Autodesk Inventor part; units mm, degrees
ref_plane "YZ Plane" through (0, 0, 0) normal (1, 0, 0) x (0, 1, 0)
ref_plane "XZ Plane" through (0, 0, 0) normal (0, 1, 0) x (-1, 0, 0)
ref_plane "XY Plane" through (0, 0, 0) normal (0, 0, 1) x (1, 0, 0)
sketch "草图1" plane through (0, 0, 0) normal (0, 0, 1) x (1, 0, 0)
  line L0 (-18, -13) -> (18, -13)
  line L1 (18, -13) -> (18, 13)
  line L2 (18, 13) -> (-18, 13)
  line L3 (-18, 13) -> (-18, -13)
  point P0 (0, 0)
  point P1 (0, 13)
  point P2 (-18, 0)
  dimension "d0" = 36
  dimension "d1" = 26
extrude "拉伸1" add sketch "草图1" along normal mid plane 60
sketch "草图2" plane through (-18, -13, -30) normal (0, -1, 0) x (1, 0, 0)
  line L0 (0, 0) -> (0, 60)
  line L1 (36, 60) -> (0, 60)
  line L2 (36, 0) -> (0, 0)
  arc A0 (20.5, -4) -> (18, -1.5) centre (18, -4) ccw
  line L3 (21.3793, -7) -> (20.5, -7)
  line L4 (20.5, -7) -> (20.5, -4)
  line L5 (23.1821, -5.866) -> (26, 0)
  arc A1 (18, -1.5) -> (15.5, -4) centre (18, -4) ccw
  line L6 (14.6207, -7) -> (15.5, -7)
  line L7 (15.5, -7) -> (15.5, -4)
  line L8 (12.8179, -5.866) -> (10, 0)
  arc A2 (21.3793, -7) -> (23.1821, -5.866) centre (21.3793, -5) ccw
  arc A3 (12.8179, -5.866) -> (14.6207, -7) centre (14.6207, -5) ccw
  point P0 (18, 30)
  point P1 (22.6373, 30)
  point P2 (0, 30)
  point P3 (18, 0)
  point P4 (18, 30)
  point P5 (0, 30)
  point P6 (18, 0)
  point P7 (10, 0)
  dimension "d6" = 5
  dimension "d9" = 2
extrude "拉伸2" add sketch "草图2" against normal blind 2
mirror "镜像1" about plane through (0, 0, 0) normal (0, 0, 1) of "拉伸2"
properties part number "DC_DC_POWER"
The listing builds one solid part. Answer for the finished solid, in the listing's coordinates (mm). A direction names the side the tool comes from. Give positions to 0.01 mm unless a question says otherwise; leave off trailing zeros. Loops run counter-clockwise (first coordinate to the right, second up) from the corner with the lowest first, then second, coordinate; pieces in that order, holes last. Notation, with made-up numbers: M 2,-1.5 L 37,-1.5 A22 cw 37,35.5 Z; hole C 63.25,43 d9. An arc over 180 degrees is marked long. One line per item, written item: value.
1. For faces 4 (the face through (0, -11, -31)), 5 (the face through (2.5, -12, -36)), 6 (the face through (0, -11, 31)), 7 (the face through (-2.5, -12, 35)), determine the directions among +Z, -Z, +X, -X, +Y, -Y from which every point of the face is accessible in a straight line to the end or side of a thin tool.
Found:
face 4: -Z, +X, -X, +Y
face 5: -Z, +Y, -Y
face 6: +Z, +X, -X, +Y
face 7: +Z, +Y, -Y
2. Each of these flat-tipped pins is pushed along its axis until it touches: P1, Ø8, axis at x = 13.5, y = -9.5, coming from the -Z side; P2, Ø2, axis at y = -12, z = 35.5, coming from the -X side; P3, Ø12, axis at x = -14, y = 8, coming from the +Z side. Where does it stop, or does it pass through?
Found:
P1: z = -30
P2: x = -5.84
P3: z = 30
3. Section C-C on x = -6 is taken. Determine the outline of the cut face in (y, z).
Found:
outline: M -13,-34.16 L -11,-34.16 L -11,-30 L 13,-30 L 13,30 L -11,30 L -11,34.16 L -13,34.16 Z
4. Section D-D on x = 11 is taken. Determine the outline of the cut face in (y, z), plus the area to 3 significant figures.
Found:
outline: M -13,-30 L 13,-30 L 13,30 L -13,30 Z
area: 1,560 mm^2
5. Section B-B on y = 0 is taken. Determine the outline of the cut face in (x, z), plus the area to 3 significant figures.
Found:
outline: M -18,-30 L 18,-30 L 18,30 L -18,30 Z
area: 2,160 mm^2
6. For a pull along X with two mould halves and no side action, classify faces 1 (the face through (2.5, -12, 35)), 2 (the face through (6.61, -12.01, 32.89)), 3 (the face through (0, 0, 30)) as pulls with the +X half, pulls with the -X half, needs draft (parallel to the pull), parting line crosses it, or undercut.
Found:
face 1: undercut
face 2: pulls with the +X half
face 3: needs draft
7. Section A-A on x = 0 is taken. Determine the outline of the cut face in (y, z).
Found:
outline: M -13,-31.5 L -11,-31.5 L -11,-30 L 13,-30 L 13,30 L -11,30 L -11,31.5 L -13,31.5 Z
8. Find the intervals of material crossed by probe 1 along Z at (x, y) = (9, 7.5); probe 2 along Y at (x, z) = (-3, -33.5), in increasing order.
Found:
probe 1: -30 to 30
probe 2: -13 to -11
